from build123d import *
from build123d.topology import SkipClean

# Parameters (mm, degrees)
SKETCH3_R           = 40
SKETCH3_R_2         = 35.480196097
BOSS_EXTRUDE1_DEPTH = 2
BOSS_EXTRUDE2_START = -2
SKETCH4_R           = 41.3
SKETCH4_R_2         = 40
BOSS_EXTRUDE2_DEPTH = 2
CUT_EXTRUDE1_DEPTH  = 10
SKETCH7_R           = 29.880196097
BOSS_EXTRUDE3_DEPTH = 0.5
BOSS_EXTRUDE4_START = 1
SKETCH8_R           = 41.3
SKETCH8_R_2         = 29.880196097
BOSS_EXTRUDE4_DEPTH = 1
SKETCH12_R          = 1.7
CUT_EXTRUDE2_DEPTH  = 60.256898333


# Read off the part's stored shape, not the designer's step: Revolve3
with BuildPart() as part:
    # Revolve3 outline → Revolve3 (revolve)
    with BuildSketch(Plane.XY):
        Polygon((35.480196097, 2), (29.880196097, 2), (27.480196097, -10), (28.5, -10), (30.5, 0), (35.480196097, 0), align=None)
    revolve(axis=Axis((0, 0, 0), (0, 1, 0)))

    # Sketch3 → Boss-Extrude1 (add)
    with BuildSketch(Plane(origin=(0, 2, 0), x_dir=(1, 0, 0), z_dir=(0, 1, 0))):
        with Locations(Location((0, 0, 0), (0, 0, 270))):
            Circle(SKETCH3_R)
        Circle(SKETCH3_R_2, mode=Mode.SUBTRACT)
    extrude(amount=-BOSS_EXTRUDE1_DEPTH)

    # Sketch4 → Boss-Extrude2 (add)
    with BuildSketch(Plane.XZ.offset(BOSS_EXTRUDE2_START)):
        with Locations(Location((0, 0, 0), (0, 0, 270))):
            Circle(SKETCH4_R)
        Circle(SKETCH4_R_2, mode=Mode.SUBTRACT)
    extrude(amount=BOSS_EXTRUDE2_DEPTH)

    # Sketch6 → Cut-Extrude1 (cut)
    with BuildSketch(Plane(origin=(0, 2, 0), x_dir=(1, 0, 0), z_dir=(0, 1, 0))):
        with BuildLine():
            ThreePointArc((41.3, 0), (41.268948935, 1.601203852), (41.175842432, 3.2))
            Line((41.175842432, 3.2), (35.5, 3.2))
            ThreePointArc((35.5, 3.2), (32.3, 0), (35.5, -3.2))
            Line((35.5, -3.2), (41.175842432, -3.2))
            ThreePointArc((41.175842432, -3.2), (41.268948935, -1.601203852), (41.3, 0))
        make_face()
        with BuildLine():
            ThreePointArc((-3.2, -41.175842432), (0, -41.3), (3.2, -41.175842432))
            Line((3.2, -41.175842432), (3.2, -35.5))
            ThreePointArc((3.2, -35.5), (0, -32.3), (-3.2, -35.5))
            Line((-3.2, -35.5), (-3.2, -41.175842432))
        make_face()
        with BuildLine():
            Line((-35.5, 3.2), (-41.175842432, 3.2))
            ThreePointArc((-41.175842432, 3.2), (-41.3, 0), (-41.175842432, -3.2))
            Line((-41.175842432, -3.2), (-35.5, -3.2))
            ThreePointArc((-35.5, -3.2), (-32.3, 0), (-35.5, 3.2))
        make_face()
        with BuildLine():
            ThreePointArc((-3.2, 35.5), (0, 32.3), (3.2, 35.5))
            Line((3.2, 35.5), (3.2, 41.175842432))
            ThreePointArc((3.2, 41.175842432), (0, 41.3), (-3.2, 41.175842432))
            Line((-3.2, 41.175842432), (-3.2, 35.5))
        make_face()
    extrude(amount=-CUT_EXTRUDE1_DEPTH, mode=Mode.SUBTRACT)

    # Sketch7 → Boss-Extrude3 (add)
    # profile 1 of 5: a face of its own
    with SkipClean():  # the faces are left unmerged after this step: merging them gives an invalid solid
        with BuildSketch(Plane(origin=(0, 2, 0), x_dir=(1, 0, 0), z_dir=(0, 1, 0))):
            with BuildLine():
                Line((41.175842432, -3.2), (35.5, -3.2))
                ThreePointArc((35.5, -3.2), (32.3, 0), (35.5, 3.2))
                Line((35.5, 3.2), (41.175842432, 3.2))
                ThreePointArc((41.175842432, 3.2), (29.203510063, 29.203510063), (3.2, 41.175842432))
                Line((3.2, 41.175842432), (3.2, 35.5))
                ThreePointArc((3.2, 35.5), (0, 32.3), (-3.2, 35.5))
                Line((-3.2, 35.5), (-3.2, 41.175842432))
                ThreePointArc((-3.2, 41.175842432), (-29.203510063, 29.203510063), (-41.175842432, 3.2))
                Line((-41.175842432, 3.2), (-35.5, 3.2))
                ThreePointArc((-35.5, 3.2), (-32.3, 0), (-35.5, -3.2))
                Line((-35.5, -3.2), (-41.175842432, -3.2))
                ThreePointArc((-41.175842432, -3.2), (-29.203510063, -29.203510063), (-3.2, -41.175842432))
                Line((-3.2, -41.175842432), (-3.2, -35.5))
                ThreePointArc((-3.2, -35.5), (0, -32.3), (3.2, -35.5))
                Line((3.2, -35.5), (3.2, -41.175842432))
                ThreePointArc((3.2, -41.175842432), (29.203510063, -29.203510063), (41.175842432, -3.2))
            make_face()
            Circle(SKETCH7_R, mode=Mode.SUBTRACT)
        # profile 2 of 5: a face of its own
        with BuildSketch(Plane(origin=(0, 2, 0), x_dir=(1, 0, 0), z_dir=(0, 1, 0))):
            with BuildLine():
                Line((-35.5, 3.2), (-41.175842432, 3.2))
                ThreePointArc((-41.175842432, 3.2), (-41.3, 0), (-41.175842432, -3.2))
                Line((-41.175842432, -3.2), (-35.5, -3.2))
                ThreePointArc((-35.5, -3.2), (-32.3, 0), (-35.5, 3.2))
            make_face()
        # profile 3 of 5: a face of its own
        with BuildSketch(Plane(origin=(0, 2, 0), x_dir=(1, 0, 0), z_dir=(0, 1, 0))):
            with BuildLine():
                ThreePointArc((-3.2, -41.175842432), (0, -41.3), (3.2, -41.175842432))
                Line((3.2, -41.175842432), (3.2, -35.5))
                ThreePointArc((3.2, -35.5), (0, -32.3), (-3.2, -35.5))
                Line((-3.2, -35.5), (-3.2, -41.175842432))
            make_face()
        # profile 4 of 5: a face of its own
        with BuildSketch(Plane(origin=(0, 2, 0), x_dir=(1, 0, 0), z_dir=(0, 1, 0))):
            with BuildLine():
                ThreePointArc((41.175842432, -3.2), (41.268948935, -1.601203852), (41.3, 0))
                ThreePointArc((41.3, 0), (41.268948935, 1.601203852), (41.175842432, 3.2))
                Line((41.175842432, 3.2), (35.5, 3.2))
                ThreePointArc((35.5, 3.2), (32.3, 0), (35.5, -3.2))
                Line((35.5, -3.2), (41.175842432, -3.2))
            make_face()
        # profile 5 of 5: a face of its own
        with BuildSketch(Plane(origin=(0, 2, 0), x_dir=(1, 0, 0), z_dir=(0, 1, 0))):
            with BuildLine():
                Line((3.2, 35.5), (3.2, 41.175842432))
                ThreePointArc((3.2, 41.175842432), (0, 41.3), (-3.2, 41.175842432))
                Line((-3.2, 41.175842432), (-3.2, 35.5))
                ThreePointArc((-3.2, 35.5), (0, 32.3), (3.2, 35.5))
            make_face()
        extrude(amount=-BOSS_EXTRUDE3_DEPTH)

    # Sketch8 → Boss-Extrude4 (add)
    with SkipClean():  # the faces are left unmerged after this step: merging them gives an invalid solid
        with BuildSketch(Plane(origin=(0, 2, 0), x_dir=(1, 0, 0), z_dir=(0, 1, 0)).offset(BOSS_EXTRUDE4_START)):
            with Locations(Location((0, 0, 0), (0, 0, 94.4438364))):
                Circle(SKETCH8_R)
            with Locations(Location((0, 0, 0), (0, 0, 270))):
                Circle(SKETCH8_R_2, mode=Mode.SUBTRACT)
        extrude(amount=-BOSS_EXTRUDE4_DEPTH)

    # Sketch12 → Cut-Extrude2 (cut, through all)
    with SkipClean():  # the faces are left unmerged after this step: merging them gives an invalid solid
        with BuildSketch(Plane.XZ):
            with Locations(Location((0, 35.5, 0), (0, 0, 270))):
                Circle(SKETCH12_R)
            with Locations(Location((35.5, 0, 0), (0, 0, 270))):
                Circle(SKETCH12_R)
            with Locations(Location((-35.5, 0, 0), (0, 0, 270))):
                Circle(SKETCH12_R)
            with Locations(Location((0, -35.5, 0), (0, 0, 270))):
                Circle(SKETCH12_R)
        extrude(amount=-CUT_EXTRUDE2_DEPTH, mode=Mode.SUBTRACT)

    # Sketch9 → Cut-Revolve2 (revolve, cut)
    with SkipClean():  # the faces are left unmerged after this step: merging them gives an invalid solid
        with BuildSketch(Plane.XY):
            Polygon((-27.480196097, -10), (-31.397991817, 9.588858549), (0, 9.588858549), (0, -10), align=None)
        revolve(axis=Axis((0, 9.588858549, 0), (0, -1, 0)), mode=Mode.SUBTRACT)


solid = part.part
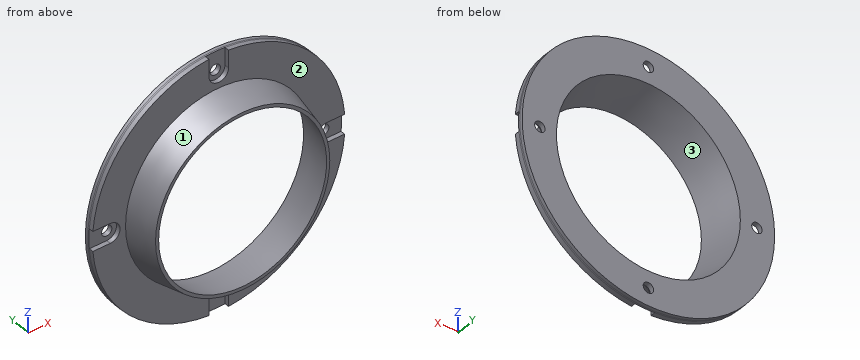
Source: CAD feature listing. Evaluate the final solid. Frame: model axes, mm. Face numbers are marked on the shaded views. Coordinates: 2 decimals unless noted, no trailing zeros. Loops run counter-clockwise (first coordinate to the right, second up) from the corner with the lowest first, then second, coordinate; pieces in that order, holes last. Notation, with made-up numbers: (51.5, 75.25) -> (93.5, 75.25) arc R12 ccw to (93.5, 87.25) -> close; hole circle Ø4 at (-12.75, 56). An arc over 180 degrees is marked (long way). Answer in a Markdown table with one row per item. Add a question column.
Q1. Contact query for flat-ended pins moving along their axis: pin 1 Ø1.6 at (x, y) = (38.5, 1) entering from +Z; pin 2 Ø2 at (x, z) = (35.5, 0) entering from +Y; pin 3 Ø1.2 at (x, y) = (-38, 0.5) entering from +Z; pin 4 Ø5 at (y, z) = (-3, 15) entering from -X. Output: stop coordinate, or through.
Q2. Section A-A on y = -3. Return the cut outline in (x, z).
Q3. Ray query, line 1 along X through (y, z) = (2.55, 0); line 2 along X through (y, z) = (-3.5, 15.5); line 3 along Z through (x, y) = (6.5, -9). Return the intervals inside material, ascending.
Q4. Pull-direction query (Z, two-part tool) for the marked faces 1, 2 and 3; classes: pulls with the +Z half, pulls with the -Z half, needs draft (parallel to the pull), parting line crosses it, or undercut.
Computed values:
| question | item | result |
|---|---|---|
| 1 | pin 1 | stops at z = 16.86 |
| 1 | pin 2 | passes through |
| 1 | pin 3 | stops at z = 17.52 |
| 1 | pin 4 | stops at x = -27.29 |
| 2 | outline | circle Ø59.8 at (0, 0); hole circle Ø57.76 at (0, 0) |
| 3 | line 1 | x = -41.3 to -37.2, -33.8 to -29.99, 29.99 to 33.8, 37.2 to 41.3 |
| 3 | line 2 | x = -25.45 to -24.25, 24.25 to 25.45 |
| 3 | line 3 | z = -27.95 to -26.91, 26.91 to 27.95 |
| 4 | face 1 | parting line crosses it |
| 4 | face 2 | needs draft |
| 4 | face 3 | undercut |
